Design review of the part built by this model. Coordinates are the model's own, in mm. Face numbers are marked on the shaded views. A direction names the side the tool comes from. Give positions to 0.01 mm unless a question says otherwise; leave off trailing zeros. Write each loop counter-clockwise with the first axis right and the second up, starting at its lowest first coordinate (ties: lowest second). Pieces come first, ordered by that corner, then holes.
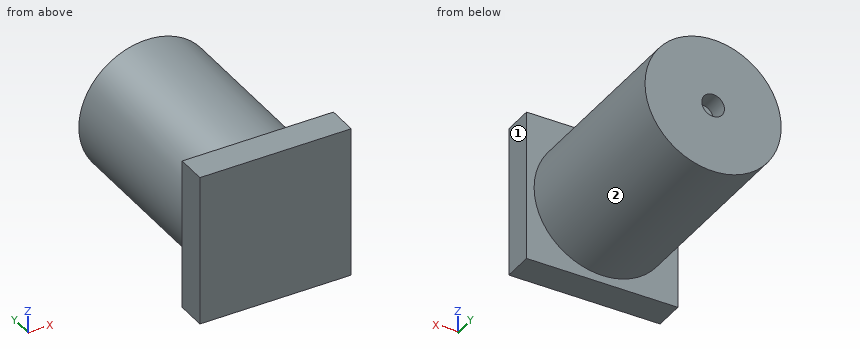
```python
from build123d import *

# Parameters (mm, degrees)
ESBO_O2_W                = 200
ESBO_O2_H                = 200
RESSALTO_EXTRUS_O1_DEPTH = 40
ESBO_O3_R                = 90
RESSALTO_EXTRUS_O2_DEPTH = 250
ESBO_O4_R                = 15
CORTE_EXTRUS_O1_DEPTH    = 25


with BuildPart() as part:
    # Esboço2 → Ressalto-extrusão1 (new body)
    with BuildSketch(Plane(origin=(0, 0, 0), x_dir=(1, 0, 0), z_dir=(0, 1, 0))):
        Rectangle(ESBO_O2_W, ESBO_O2_H)
    extrude(amount=RESSALTO_EXTRUS_O1_DEPTH)

    # Esboço3 → Ressalto-extrusão2 (add)
    with BuildSketch(Plane(origin=(0, 40, 0), x_dir=(1, 0, 0), z_dir=(0, 1, 0))):
        Circle(ESBO_O3_R)
    extrude(amount=RESSALTO_EXTRUS_O2_DEPTH)

    # Esboço4 → Corte-extrusão1 (cut)
    with BuildSketch(Plane(origin=(0, 290, 0), x_dir=(1, 0, 0), z_dir=(0, 1, 0))):
        Circle(ESBO_O4_R)
    extrude(amount=-CORTE_EXTRUS_O1_DEPTH, mode=Mode.SUBTRACT)


solid = part.part
```
(1) Tool access review of the marked faces 1 and 2: name each direction out of +Z, -Z, +X, -X, +Y, -Y from which nothing blocks a thin tool from reaching the whole face with its end or side.
Resolved:
face 1: +Z, -Z, +X, +Y, -Y
face 2: +Y
(2) Consider section B-B, the plane x = 0. Give the boundary of the cut face in (y, z).
Resolved:
outline: (0, -100) - (40, -100) - (40, -90) - (290, -90) - (290, -15) - (265, -15) - (265, 15) - (290, 15) - (290, 90) - (40, 90) - (40, 100) - (0, 100) - close
(3) To check wall thickness, follow L1, parallel to Z at x = 0, y = 281.75; L2, parallel to Y at x = 77, z = 88. State the ranges of each line that lie inside material, in increasing order.
Resolved:
L1: z = -90 to -15, 15 to 90
L2: y = 0 to 40
(4) Consider section C-C, the plane y = 187. Give the boundary of the cut face in (x, z), then the cut area to 3 significant figures.
Resolved:
outline: circle Ø180 at (0, 0)
area: 25,400 mm2
(5) Consider section D-D, the plane x = -43. Give the boundary of the cut face in (y, z).
Resolved:
outline: (0, -100) - (40, -100) - (40, -79.06) - (290, -79.06) - (290, 79.06) - (40, 79.06) - (40, 100) - (0, 100) - close
(6) Consider section A-A, the plane z = 0. Give the boundary of the cut face in (x, y), then the cut area to 4 significant figures.
Resolved:
outline: (-100, 0) - (100, 0) - (100, 40) - (90, 40) - (90, 290) - (15, 290) - (15, 265) - (-15, 265) - (-15, 290) - (-90, 290) - (-90, 40) - (-100, 40) - close
area: 52,250 mm2
(7) Clearance check with flat-ended pins moving along their axes: P1, Ø6, axis at y = 53, z = -58.5, coming from the -X side; P2, Ø3, axis at y = 185.5, z = -5, coming from the +X side; P3, Ø12, axis at x = -22, z = -11.5, coming from the -Y side; P4, Ø3, axis at y = 176, z = 20, coming from the -X side. State where each tip first meets the part, or that it passes through.
Resolved:
P1: stops at x = -70.85
P2: stops at x = 89.93
P3: stops at y = 0
P4: stops at x = -88.08
